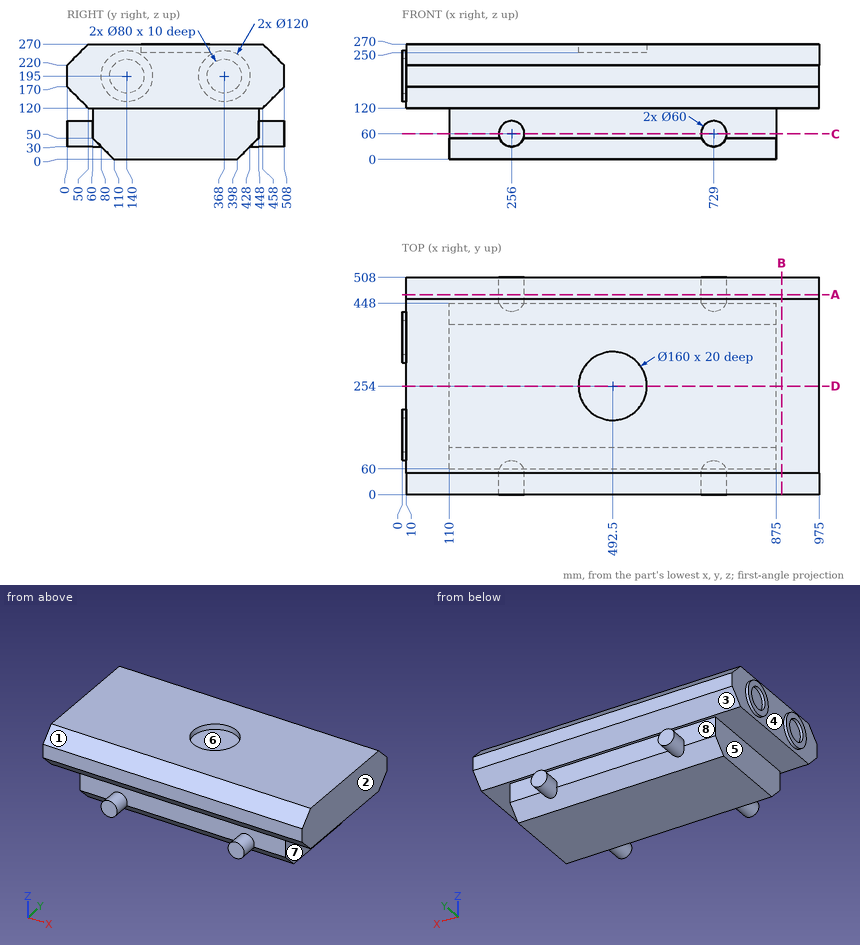
Design review of the part shown in the three views and the two pictorial views. Dimensions are in mm from the part's minimum x, y and z. A direction names the side the tool comes from. Round coordinates to 2 decimals unless told otherwise and drop trailing zeros. Write each loop counter-clockwise with the first axis right and the second up, starting at its lowest first coordinate (ties: lowest second). Pieces come first, ordered by that corner, then holes. Notation, with made-up numbers: (1.25, -7.5) - (37.25, -7.5) arc R12 ccw to (37.25, -2.5) - close; hole circle Ø11 at (-29, 68). An arc over 180 degrees is marked (long way). Return JSON: item names as keys, results as strings. Group by question number.
Item 1: We need section B-B on x = 887.5. Write out the cut boundary in (y, z).
Item 2: The part is to be moulded in two halves that separate along Z. For the marked faces 1, 2 and 3, say which applies: pulls with the +Z half, pulls with the -Z half, needs draft (parallel to the pull), parting line crosses it, or undercut.
Item 3: Machinability: for the marked faces 4, 5, 6, 7 and 8, which of the approach directions +Z, -Z, +X, -X, +Y, -Y give a long, thin tool a straight path to every point of the face, cutting with its end or side? Answer none if there is none.
Item 4: We need section C-C on z = 60. Write out the cut boundary in (x, y), and give its area (3 significant figures).
Item 5: For probe 1 along Y at (x, z) = (4.25, 195); probe 2 along X at (y, z) = (191, 48.5); probe 3 along Z at (x, y) = (81, 289), list the stretches that pass through material, from the lowest coordinate up. Write a range as [from, to].
Item 6: We need section A-A on y = 468. Write out the cut boundary in (x, z).
Item 7: We need section D-D on y = 254. Write out the cut boundary in (x, z).
Item 8: Insertion check: P1, Ø3, axis at x = 511, z = 45, coming from the +Y side; P2, Ø1.5, axis at x = 138.5, z = 105, coming from the +Y side; P3, Ø3, axis at y = 204, z = 214, coming from the -X side. Each pin has a flat end and moves straight along its axis. Give the tip position at first contact, or say it passes through.
Model answer:
{
 "1": {"outline": "(0, 170) - (50, 120) - (458, 120) - (508, 170) - (508, 220) - (458, 270) - (50, 270) - (0, 220) - close"},
 "2": {"face 1": "pulls with the +Z half", "face 2": "needs draft", "face 3": "undercut"},
 "3": {"face 4": "-X", "face 5": "-Z, -X, +Y, -Y", "face 6": "+Z", "face 7": "-Z, +X, +Y, -Y", "face 8": "+Y"},
 "4": {"outline": "(110, 60) - (226, 60) - (226, 0) - (286, 0) - (286, 60) - (699, 60) - (699, 0) - (759, 0) - (759, 60) - (875, 60) - (875, 448) - (759, 448) - (759, 508) - (699, 508) - (699, 448) - (286, 448) - (286, 508) - (226, 508) - (226, 448) - (110, 448) - close", "area": "311,000 mm²"},
 "5": {"probe 1": "y = [80, 100], [180, 200], [308, 328], [408, 428]", "probe 2": "x = [110, 875]", "probe 3": "z = [120, 270]"},
 "6": {"outline": "(10, 130) - (975, 130) - (975, 260) - (10, 260) - close; circle Ø60 at (256, 60); circle Ø60 at (729, 60)"},
 "7": {"outline": "(10, 120) - (110, 120) - (110, 0) - (875, 0) - (875, 120) - (975, 120) - (975, 270) - (572.5, 270) - (572.5, 250) - (412.5, 250) - (412.5, 270) - (10, 270) - close"},
 "8": {"P1": "stops at y = 444.5", "P2": "stops at y = 448", "P3": "stops at x = 10"}
}
